Autodesk Inventor part; units mm, degrees
ref_plane "YZ Plane" through (0, 0, 0) normal (1, 0, 0) x (0, 1, 0)
ref_plane "XZ Plane" through (0, 0, 0) normal (0, 1, 0) x (-1, 0, 0)
ref_plane "XY Plane" through (0, 0, 0) normal (0, 0, 1) x (1, 0, 0)
sketch "Sketch1" plane through (0, 0, 0) normal (0, 0, 1) x (1, 0, 0)
  line L0 (0, 0) -> (50, 0)
  line L1 (50, 0) -> (50, 52.5)
  line L2 (50, 52.5) -> (0, 52.5)
  line L3 (0, 52.5) -> (0, 0)
  dimension "d0" = 50
  dimension "d1" = 52.5
extrude "Extrusion1" add sketch "Sketch1" along normal blind 3
sketch "Sketch2" plane through (0, 0, 3) normal (0, 0, 1) x (1, 0, 0)
  line L0 (2, 50.5) -> (48, 50.5)
  line L1 (48, 50.5) -> (48, 2)
  line L2 (48, 2) -> (2, 2)
  line L3 (2, 2) -> (2, 50.5)
  dimension "d4" = 46
  dimension "d5" = 48.5
extrude "Extrusion2" cut sketch "Sketch2" against normal blind 10
sketch "Sketch3" plane through (0, 0, 3) normal (0, 0, 1) x (1, 0, 0)
  line L0 (48, 2) -> (2, 2)
  line L1 (0, 52.5) -> (0, 0)
  line L2 (2, 2) -> (0, 2)
  line L3 (0, 2) -> (0, 0)
  line L4 (0, 0) -> (2, 0)
  line L5 (2, 0) -> (2, 2)
  line L6 (0, 0) -> (50, 0)
  line L7 (13.7, 2) -> (15.7, 2)
  line L8 (15.7, 2) -> (15.7, 0)
  line L9 (15.7, 0) -> (13.7, 0)
  line L10 (13.7, 0) -> (13.7, 2)
  line L11 (0, 2) -> (2, 2)
  line L12 (2, 2) -> (2, 0)
  line L13 (2, 0) -> (0, 0)
  line L14 (0, 0) -> (0, 2)
  line L15 (13.7, 2) -> (15.7, 2)
  line L16 (15.7, 2) -> (15.7, 0)
  line L17 (15.7, 0) -> (13.7, 0)
  line L18 (13.7, 0) -> (13.7, 2)
  dimension "d8" = 2
  dimension "d9" = 11.7
extrude "Extrusion3" add sketch "Sketch3" along normal blind 87.5 contours L8 L6 L10 L0 | L5 L4 L1 L2
chamfer "Chamfer1" distance 2 angle 60 1 edges at (1, 2, 90.5) measured on face at (1.3333, 0.6667, 90.5)
chamfer "Chamfer2" distance 2 angle 60 1 edges at (14.7, 2, 90.5) measured on face at (14.3667, 0.6667, 90.5)
sketch "Sketch4" plane through (0, 0, 0) normal (0, -1, 0) x (1, 0, 0)
  line L0 (0, 0) -> (50, 0)
  line L1 (0, 0) -> (0, 90.5)
  line L2 (12.85, 1.5) -> (2.85, 1.5)
  line L3 (2.85, 1.5) -> (2.85, 2.5)
  line L4 (2.85, 2.5) -> (12.85, 2.5)
  line L5 (12.85, 2.5) -> (12.85, 1.5)
  dimension "d18" = 10
  dimension "d19" = 1
  dimension "d20" = 1.5
  dimension "d21" = 2.85
extrude "Extrusion4" cut sketch "Sketch4" against normal blind 10
sketch "Sketch5" plane through (0, 0, 0) normal (0, -1, 0) x (1, 0, 0)
  line L0 (12.85, 2.5) -> (12.85, 1.5)
  line L1 (2.85, 1.5) -> (2.85, 2.5)
  line L2 (0, 0) -> (50, 0)
  line L3 (14.1, 2.5) -> (14.966, 2)
  line L4 (14.966, 2) -> (14.1, 1.5)
  line L5 (14.1, 1.5) -> (14.1, 2.5)
  line L6 (2, 3) -> (48, 3)
  line L7 (2, 2.8) -> (0.2, 2.8)
  line L8 (0.2, 2.8) -> (0.2, 0.2)
  line L9 (0.2, 0.2) -> (2, 0.2)
  line L10 (2, 0.2) -> (2, 2.8)
  line L11 (2, 3) -> (13.7, 3)
  dimension "d24" = 1
  dimension "d25" = 1.8
  dimension "d26" = 0.85
  dimension "d27" = 1.25
  dimension "d28" = 1.8
  dimension "d29" = 2.6
  dimension "d30" = 2.6
  dimension "d31" = 1
  dimension "d32" = 1
  dimension "d33" = 0.5
  dimension "d103" = 0.2
  dimension "d104" = 0.2
extrude "Extrusion5" add sketch "Sketch5" along normal blind 4
sketch "Sketch6" plane through (0, 52.5, 0) normal (0, 1, 0) x (1, 0, 0)
  line L0 (0, 0) -> (0, -3)
  line L1 (50, -3) -> (0, -3)
  line L2 (12.66, -1.75) -> (12.66, -2.77)
  line L3 (12.66, -2.77) -> (2, -2.77)
  line L4 (2, -2.77) -> (2, -0.23)
  line L5 (2, -0.23) -> (12.66, -0.23)
  line L6 (12.66, -0.23) -> (12.66, -2.77)
  line L7 (50, 0) -> (0, 0)
  point P0 (2.85, -1.5)
  dimension "d1" = 52.5
  dimension "d51" = 10.66
  dimension "d52" = 2.54
  dimension "d54" = 0.23
  dimension "d55" = 2
  dimension "d57" = 0.23
extrude "Extrusion6" cut sketch "Sketch6" against normal blind 4
sketch "Sketch7" plane through (2, 50.5, 3) normal (0, -1, 0) x (1, 0, 0)
  line L0 (10.66, -2.77) -> (0, -2.77)
  line L1 (46, -3) -> (0, -3)
  line L2 (11, -3) -> (0, -3)
  line L3 (0, -3) -> (0, -2.77)
  line L4 (0, 0) -> (11, 0)
  line L5 (0, -0.23) -> (0, 0)
  line L6 (11, 0) -> (11, -3)
  line L7 (10.66, -2.77) -> (0, -2.77)
  line L8 (0, -0.23) -> (10.66, -0.23)
  line L9 (48, 0) -> (-2, 0)
  line L10 (10.66, -2.77) -> (10.66, -0.23)
  line L11 (11, -3) -> (11, 0)
  line L12 (10.66, -2.77) -> (10.66, -0.23)
  line L13 (10.66, -2.77) -> (10.66, -0.23)
  point P0 (-2, -3)
extrude "Extrusion7" add sketch "Sketch7" along normal blind 6.5
sketch "Sketch8" plane through (0, 52.5, 0) normal (0, 1, 0) x (1, 0, 0)
  line L0 (50, 0) -> (0, 0)
  line L1 (50, 0) -> (50, -3)
  line L2 (12.8966, -0.5) -> (14.6286, -1.5)
  line L3 (12.8966, -0.5) -> (14.8966, -0.5) construction
  line L4 (14.6286, -1.5) -> (12.8966, -2.5)
  line L5 (12.66, -2.77) -> (12.66, -0.23)
  line L6 (12.8966, -2.5) -> (12.8966, -0.5)
  line L7 (13.0189, -2.1236) -> (13.0189, -0.9087)
  line L8 (13.0189, -0.9087) -> (13.0189, -0.7479)
  line L9 (13.0189, -0.7479) -> (14.3309, -1.5054)
  line L10 (13.0189, -2.1236) -> (13.0189, -2.2521)
  line L11 (13.0189, -2.2521) -> (14.3309, -1.5054)
  dimension "d60" = 2
  dimension "d61" = 30
  dimension "d62" = 2
  dimension "d63" = 60
  dimension "d64" = 0.5
  dimension "d65" = 35.3714
  dimension "d98" = 1.312
  dimension "d99" = 0.1535
  dimension "d100" = 0.1535
sketch "Sketch9" plane through (0, 52.5, 0) normal (0, 1, 0) x (1, 0, 0)
  line L0 (50, 0) -> (0, 0)
  line L1 (0, 0) -> (0, -3)
  line L2 (50, -3) -> (0, -3)
  line L3 (2, -2.77) -> (2, -0.23)
  line L4 (2, -3) -> (0, -3)
  line L5 (0, -3) -> (0, 0)
  line L6 (0, 0) -> (2, 0)
  line L7 (2, 0) -> (2, -3)
  line L8 (1.75, -2.5) -> (0.25, -2.5)
  line L9 (0.25, -2.5) -> (0.25, -0.5)
  line L10 (0.25, -0.5) -> (1.75, -0.5)
  line L11 (1.75, -0.5) -> (1.75, -2.5)
  dimension "d74" = 2
  dimension "d75" = 3
  dimension "d76" = 0
  dimension "d77" = 0
  dimension "d78" = 0
  dimension "d79" = 0
  dimension "d81" = 1.5
  dimension "d82" = 2
  dimension "d94" = 0.5
  dimension "d95" = 0.25
extrude "Extrusion10" add sketch "Sketch9" along normal blind 4
extrude "Extrusion11" add sketch "Sketch8" along normal blind 4
properties part number "Zijplaat 1"
Design review of the part built by this model. Coordinates are the model's own, in mm. A direction names the side the tool comes from. Coordinates: 2 decimals unless noted, no trailing zeros. Loops run counter-clockwise (first coordinate to the right, second up) from the corner with the lowest first, then second, coordinate; pieces in that order, holes last.
Item 1: For faces 4 (the flat face through (1.75, 54, 1)), 5 (the flat face through (1, -2, 0.2)), 6 (the flat face through (30, 50.5, 2)), 7 (the flat face through (8, 1, 3)), list the 3-axis set-ups (+Z, -Z, +X, -X, +Y, -Y) from which the entire face can be reached by the end or side of a thin tool; tool diameter is ignored.
Completed:
face 4: +Y
face 5: -Z, +X, -X, -Y
face 6: +Z, -Z
face 7: +Z, +Y, -Y
Item 2: Clearance check with flat-ended pins moving along their axes: pin 1 (0.6 mm diameter, centred on y = 54.5, z = 1.5, fed in from -X); pin 2 (4 mm diameter, centred on x = 17, z = 55, fed in from +Y); pin 3 (4 mm diameter, centred on x = 7.5, y = 48, fed in from +Z); pin 4 (0.8 mm diameter, centred on y = -1.5, z = 2, fed in from -X). State where each tip first meets the part, or that it passes through.
Completed:
pin 1: stops at x = 0
pin 2: stops at y = 2
pin 3: stops at z = 3
pin 4: stops at x = 0.2
Item 3: Add section B-B (x = 37). Write out the cut boundary in (y, z), and give its area (3 significant figures).
Completed:
outline: (0, 0) - (2, 0) - (2, 3) - (0, 3) - close; (50.5, 0) - (52.5, 0) - (52.5, 3) - (50.5, 3) - close
area: 12.0 mm2
Item 4: Wall thickness on L1, parallel to Y at x = 15.5, z = 86: over which ranges is the line inside the solid? List them lowest first.
Completed:
L1: y = 0 to 2
Item 5: Draft analysis for pull direction Z (two halves, no side actions). For faces 1 (the flat face through (15.7, 1, 46)), 2 (the flat face through (8, 1, 1.5)), 3 (the flat face through (1, -2, 2.8)), state which applies: pulls with the +Z half, pulls with the -Z half, needs draft (parallel to the pull), parting line crosses it, or undercut.
Completed:
face 1: needs draft
face 2: undercut
face 3: pulls with the +Z half
Item 6: Add section D-D (x = 5). Write out the cut boundary in (y, z), and give its area (3 significant figures).
Completed:
outline: (0, 0) - (2, 0) - (2, 1.5) - (0, 1.5) - close; (0, 2.5) - (2, 2.5) - (2, 3) - (0, 3) - close; (44, 0) - (52.5, 0) - (52.5, 0.23) - (44, 0.23) - close; (44, 2.77) - (52.5, 2.77) - (52.5, 3) - (44, 3) - close
area: 7.91 mm2
Item 7: Add section C-C (z = 62). Write out the cut boundary in (x, y), and give its area (3 significant figures).
Completed:
outline: (0, 0) - (2, 0) - (2, 2) - (0, 2) - close; (13.7, 0) - (15.7, 0) - (15.7, 2) - (13.7, 2) - close
area: 8.00 mm2
Item 8: Add section A-A (y = 48). Write out the cut boundary in (x, z).
Completed:
outline: (0, 0) - (13, 0) - (13, 3) - (0, 3) - close; (48, 0) - (50, 0) - (50, 3) - (48, 3) - close; hole (2, 0.23) - (12.66, 0.23) - (12.66, 2.77) - (2, 2.77) - close
